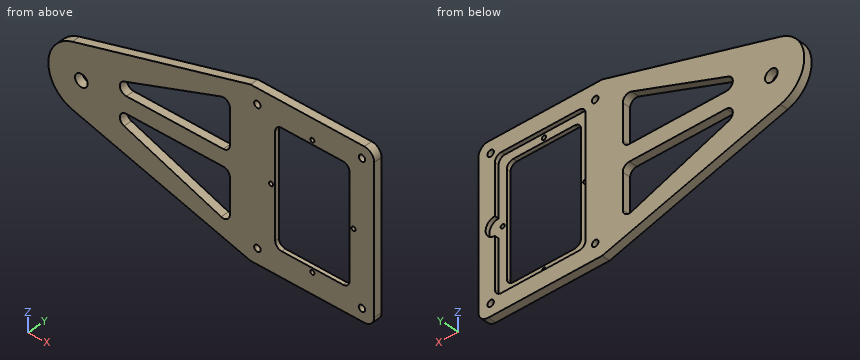
from build123d import *

# Parameters (mm, degrees)
SKETCH1_W           = 95.25
SKETCH1_H           = 127
BOSS_EXTRUDE1_DEPTH = 6.35
BOSS_EXTRUDE3_DEPTH = 6.35
SKETCH5_R           = 4.826
CUT_EXTRUDE1_DEPTH  = 213.985474857
CUT_EXTRUDE2_DEPTH  = 213.985474857
FILLET9_R           = 5
SKETCH7_R           = 5.453804141
BOSS_EXTRUDE4_DEPTH = 6.35
SKETCH8_W           = 69.85
SKETCH8_H           = 101.6
CUT_EXTRUDE3_DEPTH  = 3.175
SKETCH9_W           = 57.15
SKETCH9_H           = 88.9
CUT_EXTRUDE4_DEPTH  = 213.914467862
SKETCH11_R          = 1.5875
CUT_EXTRUDE6_DEPTH  = 213.914467862
CUT_EXTRUDE7_DEPTH  = 3.175
FILLET10_R          = 5
FILLET11_R          = 5
FILLET12_R          = 7.62
SKETCH13_R          = 2.4892
CUT_EXTRUDE8_DEPTH  = 213.985474857


with BuildPart() as part:
    # Sketch1 → Boss-Extrude1 (new body)
    with BuildSketch(Plane(origin=(0, 0, 0), x_dir=(1, 0, 0), z_dir=(0, 1, 0))):
        Rectangle(SKETCH1_W, SKETCH1_H)
    extrude(amount=BOSS_EXTRUDE1_DEPTH)

    # Sketch4 → Boss-Extrude3 (add)
    with BuildSketch(Plane(origin=(0, 6.35, 0), x_dir=(1, 0, 0), z_dir=(0, 1, 0))):
        with BuildLine():
            Line((-47.625, 63.5), (-184.759922998, 24.427842145))
            ThreePointArc((-184.759922998, 24.427842145), (-203.2, 0), (-184.759922998, -24.427842145))
            Line((-184.759922998, -24.427842145), (-47.625, -63.5))
            Line((-47.625, -63.5), (-47.625, 63.5))
        make_face()
    extrude(amount=-BOSS_EXTRUDE3_DEPTH)

    # Sketch5 → Cut-Extrude1 (cut, through all)
    with BuildSketch(Plane(origin=(0, 6.35, 0), x_dir=(1, 0, 0), z_dir=(0, 1, 0))):
        with Locations(Location((-177.8, 0, 0), (0, 0, 270))):
            Circle(SKETCH5_R)
        with Locations(Location((-22.225, 0, 0), (0, 0, 270))):
            Circle(SKETCH5_R)
    extrude(amount=-CUT_EXTRUDE1_DEPTH, mode=Mode.SUBTRACT)

    # Sketch6 → Cut-Extrude2 (cut, through all)
    with BuildSketch(Plane(origin=(0, 6.35, 0), x_dir=(1, 0, 0), z_dir=(0, 1, 0))):
        Polygon((-63.5, 45.771509083), (-171.45, 6.35), (-63.5, 6.35), align=None)
        Polygon((-63.5, -6.35), (-63.5, -45.771509083), (-171.45, -6.35), align=None)
    extrude(amount=-CUT_EXTRUDE2_DEPTH, mode=Mode.SUBTRACT)

    # Fillet9
    fillet9_edges = [part.edges().sort_by_distance(p)[0] for p in [
        (-63.5, 3.175, -45.771509083),
        (-63.5, 3.175, -6.35),
        (-171.45, 3.175, -6.35),
        (-171.45, 3.175, 6.35),
        (-63.5, 3.175, 6.35),
        (-63.5, 3.175, 45.771509083),
    ]]
    fillet(fillet9_edges, radius=FILLET9_R)

    # Sketch7 → Boss-Extrude4 (add)
    with BuildSketch(Plane(origin=(0, 6.35, 0), x_dir=(1, 0, 0), z_dir=(0, 1, 0))):
        with Locations((-22.225, 0)):
            Circle(SKETCH7_R)
    extrude(amount=-BOSS_EXTRUDE4_DEPTH)

    # Sketch8 → Cut-Extrude3 (cut)
    with BuildSketch(Plane(origin=(0, 6.35, 0), x_dir=(1, 0, 0), z_dir=(0, 1, 0))):
        Rectangle(SKETCH8_W, SKETCH8_H)
    extrude(amount=-CUT_EXTRUDE3_DEPTH, mode=Mode.SUBTRACT)

    # Sketch9 → Cut-Extrude4 (cut, through all)
    with BuildSketch(Plane(origin=(0, 3.175, 0), x_dir=(1, 0, 0), z_dir=(0, 1, 0))):
        Rectangle(SKETCH9_W, SKETCH9_H)
    extrude(amount=-CUT_EXTRUDE4_DEPTH, mode=Mode.SUBTRACT)

    # Sketch11 → Cut-Extrude6 (cut, through all)
    with BuildSketch(Plane(origin=(0, 3.175, 0), x_dir=(1, 0, 0), z_dir=(0, 1, 0))):
        with Locations(Location((-31.75, 0, 0), (0, 0, 270))):
            Circle(SKETCH11_R)
        with Locations(Location((31.75, 0, 0), (0, 0, 90))):
            Circle(SKETCH11_R)
        with Locations(Location((0, 47.625, 0), (0, 0, 270))):
            Circle(SKETCH11_R)
        with Locations(Location((0, -47.625, 0), (0, 0, 90))):
            Circle(SKETCH11_R)
    extrude(amount=-CUT_EXTRUDE6_DEPTH, mode=Mode.SUBTRACT)

    # Sketch12 → Cut-Extrude7 (cut)
    with BuildSketch(Plane(origin=(0, 6.35, 0), x_dir=(1, 0, 0), z_dir=(0, 1, 0))):
        with BuildLine():
            Line((34.925, 7.112), (34.925, -7.112))
            ThreePointArc((34.925, -7.112), (42.037, 0), (34.925, 7.112))
        make_face()
    extrude(amount=-CUT_EXTRUDE7_DEPTH, mode=Mode.SUBTRACT)

    # Fillet10
    fillet10_edges = [part.edges().sort_by_distance(p)[0] for p in [
        (-34.925, 4.7625, -50.8),
        (34.925, 4.7625, -50.8),
        (34.925, 4.7625, 50.8),
        (-34.925, 4.7625, 50.8),
    ]]
    fillet(fillet10_edges, radius=FILLET10_R)

    # Fillet11
    fillet11_edges = [part.edges().sort_by_distance(p)[0] for p in [
        (-28.575, 1.5875, 44.45),
        (-28.575, 1.5875, -44.45),
        (28.575, 1.5875, -44.45),
        (28.575, 1.5875, 44.45),
    ]]
    fillet(fillet11_edges, radius=FILLET11_R)

    # Fillet12
    fillet12_edges = [part.edges().sort_by_distance(p)[0] for p in [
        (47.625, 3.175, 63.5),
        (47.625, 3.175, -63.5),
    ]]
    fillet(fillet12_edges, radius=FILLET12_R)

    # Sketch13 → Cut-Extrude8 (cut, through all)
    with BuildSketch(Plane(origin=(0, 6.35, 0), x_dir=(1, 0, 0), z_dir=(0, 1, 0))):
        with Locations(Location((-42.286053483, 51.811053483, 0), (0, 0, 270))):
            Circle(SKETCH13_R)
        with Locations(Location((-42.286053483, -51.811053483, 0), (0, 0, 270))):
            Circle(SKETCH13_R)
        with Locations(Location((38.202339924, -54.077339924, 0), (0, 0, 270))):
            Circle(SKETCH13_R)
        with Locations(Location((38.202339924, 54.077339924, 0), (0, 0, 270))):
            Circle(SKETCH13_R)
    extrude(amount=-CUT_EXTRUDE8_DEPTH, mode=Mode.SUBTRACT)


solid = part.part
Can you work these out from the model? Positions are in its coordinate system, mm. Round coordinates to 2 decimals unless told otherwise and drop trailing zeros. Write each loop counter-clockwise with the first axis right and the second up, starting at its lowest first coordinate (ties: lowest second). Pieces come first, ordered by that corner, then holes. Notation, with made-up numbers: (7.25, 68) - (27.25, 68) arc R15 cw to (27.25, 73) - close; hole circle Ø8 at (-21, 61). An arc over 180 degrees is marked (long way). Write each question's results on one line, items separated by ' | '. Start each with the question number.
1) Suppose I cut it at C-C (z = -31). List the corners of the cut face in (x, y) for me (3 decimals).
2) Please list where these lines run through material, in increasing order: line 1 (X direction, y = 2.3, z = 0) (1 decimal); line 2 (Z direction, x = -120, y = 1.25); line 3 (X direction, y = 1.5, z = 10.5) (3 decimals).
3) Suppose I cut it at A-A (z = 21.5). List the corners of the cut face in (x, y) for me (3 decimals).
4) Suppose I cut it at B-B (x = -132). List the corners of the cut face in (y, z) for me, and give its area (3 significant figures).
5) For pin 1 Ø5 at (x, z) = (0, 47.625) entering from +Y (3 decimals); pin 2 Ø1.6 at (y, z) = (1, 18) entering from -X, each with a flat end and sliding along its axis, tell me the tip position at first contact or that it passes through.
6) Suppose I cut it at D-D (y = 2). Give the number of separate pieces and of enclosed holes in the cut face, and give its area (3 significant figures).
Here are the results:
1) outline: (-161.693, 0) - (-103.95, 0) - (-103.95, 6.35) - (-161.693, 6.35) - close; (-63.5, 0) - (-28.575, 0) - (-28.575, 3.175) - (-34.925, 3.175) - (-34.925, 6.35) - (-63.5, 6.35) - close; (28.575, 0) - (47.625, 0) - (47.625, 6.35) - (34.925, 6.35) - (34.925, 3.175) - (28.575, 3.175) - close
2) line 1: x = -203.2 to -182.6, -173 to -33.3, -30.2 to -28.6, 28.6 to 30.2, 33.3 to 47.6 | line 2: z = -42.88 to -25.14, -6.35 to 6.35, 25.14 to 42.88 | line 3: x = -200.928 to -148.109, -63.573 to -28.575, 28.575 to 47.625
3) outline: (-191.324, 0) - (-129.964, 0) - (-129.964, 6.35) - (-191.324, 6.35) - close; (-63.5, 0) - (-28.575, 0) - (-28.575, 3.175) - (-34.925, 3.175) - (-34.925, 6.35) - (-63.5, 6.35) - close; (28.575, 0) - (47.625, 0) - (47.625, 6.35) - (34.925, 6.35) - (34.925, 3.175) - (28.575, 3.175) - close
4) outline: (0, -39.46) - (6.35, -39.46) - (6.35, -20.76) - (0, -20.76) - close; (0, -6.35) - (6.35, -6.35) - (6.35, 6.35) - (0, 6.35) - close; (0, 20.76) - (6.35, 20.76) - (6.35, 39.46) - (0, 39.46) - close | area: 318 mm2
5) pin 1: stops at y = 3.175 | pin 2: stops at x = -196.49
6) separate pieces: 1 | enclosed holes: 12 | area: 15,500 mm2
